Source: three-view drawing plus pictorial views. Frame: mm from the lowest corner of the part. A direction names the side the tool comes from. Give positions to 0.01 mm unless a question says otherwise; leave off trailing zeros. Write each loop counter-clockwise with the first axis right and the second up, starting at its lowest first coordinate (ties: lowest second). Pieces come first, ordered by that corner, then holes.
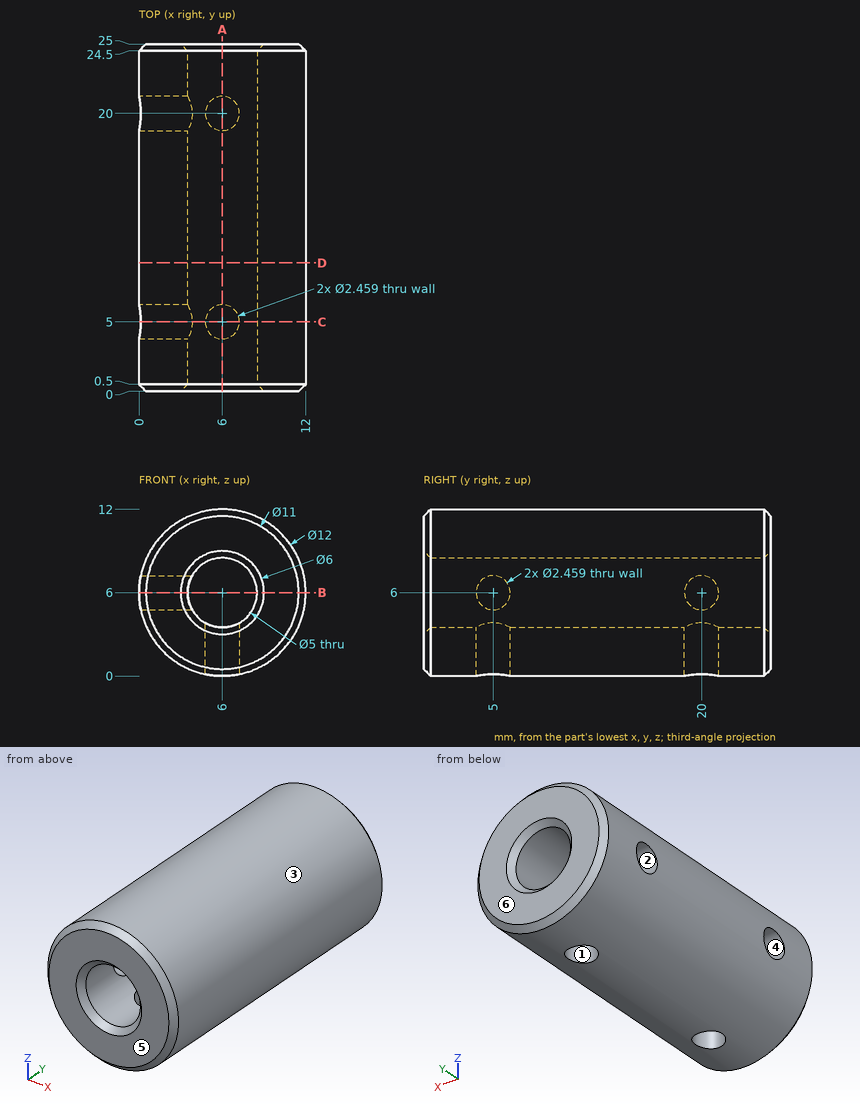
Q1. Section B-B on z = 6. Output: boundary loops of the cut face in (x, y).
Filled sheet:
outline: (0, 0.5) - (0.5, 0) - (3, 0) - (3.5, 0.5) - (3.5, 3.77) - (0, 3.77) - close; (0, 6.23) - (3.5, 6.23) - (3.5, 18.77) - (0, 18.77) - close; (0, 21.23) - (3.5, 21.23) - (3.5, 24.5) - (3, 25) - (0.5, 25) - (0, 24.5) - close; (8.5, 0.5) - (9, 0) - (11.5, 0) - (12, 0.5) - (12, 24.5) - (11.5, 25) - (9, 25) - (8.5, 24.5) - close
Q2. Section A-A on x = 6. Output: boundary loops of the cut face in (y, z).
Filled sheet:
outline: (0, 0.5) - (0.5, 0) - (3.77, 0) - (3.77, 3.5) - (0.5, 3.5) - (0, 3) - close; (0, 9) - (0.5, 8.5) - (24.5, 8.5) - (25, 9) - (25, 11.5) - (24.5, 12) - (0.5, 12) - (0, 11.5) - close; (6.23, 0) - (18.77, 0) - (18.77, 3.5) - (6.23, 3.5) - close; (21.23, 0) - (24.5, 0) - (25, 0.5) - (25, 3) - (24.5, 3.5) - (21.23, 3.5) - close
Q3. Section D-D on y = 9.25. Output: boundary loops of the cut face in (x, z), plus the area to 3 significant figures.
Filled sheet:
outline: circle Ø12 at (6, 6); hole circle Ø5 at (6, 6)
area: 93.5 mm2
Q4. Access query for the marked faces 1, 2 and 3. Directions: +Z, -Z, +X, -X, +Y, -Y. A direction counts if a zero-diameter tool reaches every point of the face in a straight line with its end or side. Return the directions, or none.
Filled sheet:
face 1: -Z
face 2: -X
face 3: +Y, -Y
Q5. Ray query, line 1 along Y through (x, z) = (6, 1.5); line 2 along Y through (x, z) = (6.5, 3.25); line 3 along Z through (x, y) = (6, 12.75). Return the intervals inside material, ascending.
Filled sheet:
line 1: y = 0 to 3.77, 6.23 to 18.77, 21.23 to 25
line 2: y = 0.2 to 3.88, 6.12 to 18.88, 21.12 to 24.8
line 3: z = 0 to 3.5, 8.5 to 12
Q6. Pin query (flat end, axial travel): P1, Ø5, axis at y = 6, z = 4, coming from the +X side; P2, Ø1, axis at x = 4.5, y = 15.5, coming from the -Z side; P3, Ø3, axis at x = 8.5, y = 4, coming from the +Z side; P4, Ø4.5, axis at x = 6, z = 6, coming from the -Y side. Return the tip coordinate at first contact, or that it passes through.
Filled sheet:
P1: stops at x = 12
P2: stops at z = 0.08
P3: stops at z = 11.92
P4: passes through
Q7. Pull-direction query (Y, two-part tool) for the marked faces 4, 5 and 6; classes: released by +Y, released by -Y, zero draft, split by the parting line, or undercut.
Filled sheet:
face 4: undercut
face 5: released by -Y
face 6: released by +Y
Q8. Section C-C on y = 5. Output: boundary loops of the cut face in (x, z), plus the area to 3 significant figures.
Filled sheet:
outline: (0.13, 4.77) arc R6 ccw to (4.77, 0.13) - (4.77, 3.82) arc R2.5 cw to (3.82, 4.77) - close; (0.13, 7.23) - (3.82, 7.23) arc R2.5 cw (long way) to (7.23, 3.82) - (7.23, 0.13) arc R6 ccw (long way) to start
area: 75.9 mm2
